from build123d import *

# Parameters (mm, degrees)
SKETCH003_R             = 23.15
PAD002_DEPTH            = 5
SKETCH004_R             = 25
PAD003_DEPTH            = 3
CHAMFER002_SIZE         = 2
SKETCH005_R             = 22
POCKET001_DEPTH         = 6
CHAMFER003_SIZE         = 2
SKETCH006_R             = 2.775
SKETCH006_R_2           = 3.5
POCKET002_DEPTH         = 5
BODY001_PLACEMENT_ANGLE = 180


with BuildPart() as part:
    # Sketch003 → Pad002 (new body)
    with BuildSketch(Plane.XY):
        Circle(SKETCH003_R)
    extrude(amount=PAD002_DEPTH)

    # Sketch004 (on Face3 of Pad002) → Pad003 (join)
    with BuildSketch(Plane.XY.offset(5)):
        Circle(SKETCH004_R)
    extrude(amount=PAD003_DEPTH)

    # Chamfer002
    chamfer002_edges = [part.edges().sort_by_distance(p)[0] for p in [
        (-25, 0, 8),
    ]]
    chamfer(chamfer002_edges, length=CHAMFER002_SIZE)

    # Sketch005 (on Face6 of Chamfer002) → Pocket001 (cut)
    with BuildSketch(Plane(origin=(0, 0, 0), x_dir=(1, 0, 0), z_dir=(0, 0, -1))):
        Circle(SKETCH005_R)
    extrude(amount=-POCKET001_DEPTH, mode=Mode.SUBTRACT)

    # Chamfer003
    chamfer003_edges = [part.edges().sort_by_distance(p)[0] for p in [
        (-22, 0, 6),
    ]]
    chamfer(chamfer003_edges, length=CHAMFER003_SIZE)

    # Sketch006 (on Face9 of Chamfer003) → Pocket002 (cut)
    with BuildSketch(Plane.XY.offset(8)):
        with Locations((0, 10)):
            Circle(SKETCH006_R)
        with Locations((0, -10)):
            Circle(SKETCH006_R_2)
    extrude(amount=-POCKET002_DEPTH, mode=Mode.SUBTRACT)


with BuildPart() as part_1:
    # Body001 placement: moved
    add(part.part.moved(Location((0, 0, -195))).rotate(Axis((0, 0, -195), (0, 1, 0)), BODY001_PLACEMENT_ANGLE))


solid = part_1.part
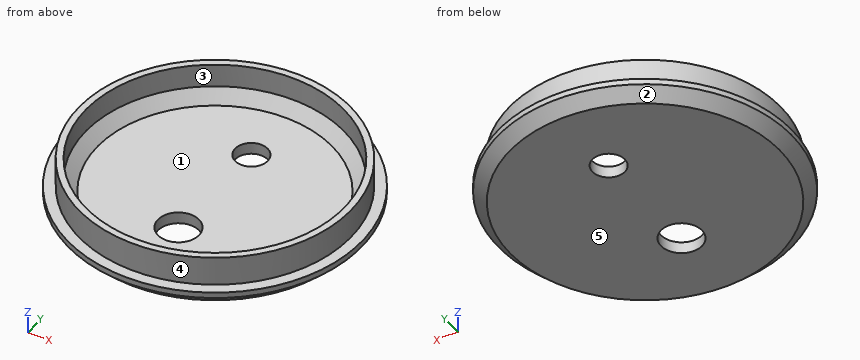
For this review, take the finished solid that the model builds, in its own axes (mm). Face numbers are marked on the shaded views. A direction names the side the tool comes from. Round coordinates to 2 decimals unless told otherwise and drop trailing zeros. Order: outer loops, then holes, each group sorted by start corner. A loop starts at its lowest first (then second) coordinate and runs counter-clockwise, first axis right, second up. Notation, with made-up numbers: (-38.5, 55.25) -> (-27.5, 55.25) arc R9 cw to (-27.5, 62.25) -> close; hole circle Ø10 at (-4.75, 88.25). An arc over 180 degrees is marked (long way). Put each result on its own line as item: value.
Q1. Add section C-C on z = -202. Write out the cut boundary in (x, y) (3 decimals).
Check result:
outline: circle Ø48 at (0, 0); hole circle Ø7 at (0, -10); hole circle Ø5.55 at (0, 10)
Q2. For probe 1 along Y at (x, z) = (0, -201.45) (3 decimals); probe 2 along Y at (x, z) = (0, -196.6); probe 3 along Y at (x, z) = (-12, -199.25), list the stretches that pass through material, from the lowest coordinate up. Write a range as [from, to].
Check result:
probe 1: [-24.55, -13.5], [-6.5, 7.225], [12.775, 24.55]
probe 2: [-23.15, -22], [22, 23.15]
probe 3: [-19.8, -18.14], [18.14, 19.8]
Q3. Insertion check: pin 1 Ø3 at (y, z) = (-1, -196.5) entering from -X; pin 2 Ø1.5 at (y, z) = (-15, -197) entering from -X; pin 3 Ø4 at (x, y) = (11, 8.5) entering from +Z. Each pin has a flat end and moves straight along its axis. Give the tip position at first contact, or say it passes through.
Check result:
pin 1: x = -23.15
pin 2: x = -18.24
pin 3: z = -201
Q4. Add section A-A on x = 0. Write out the cut boundary in (y, z) (3 decimals).
Check result:
outline: (-25, -201) -> (-23, -203) -> (-13.5, -203) -> (-13.5, -201) -> (-20, -201) -> (-22, -199) -> (-22, -195) -> (-23.15, -195) -> (-23.15, -200) -> (-25, -200) -> close; (-6.5, -203) -> (7.225, -203) -> (7.225, -201) -> (-6.5, -201) -> close; (12.775, -203) -> (23, -203) -> (25, -201) -> (25, -200) -> (23.15, -200) -> (23.15, -195) -> (22, -195) -> (22, -199) -> (20, -201) -> (12.775, -201) -> close
Q5. Add section D-D on z = -198. Write out the cut boundary in (x, y).
Check result:
outline: circle Ø46.3 at (0, 0); hole circle Ø44 at (0, 0)
Q6. Add section B-B on y = 0. Write out the cut boundary in (x, z), plus the area to 4 significant figures.
Check result:
outline: (-25, -201) -> (-23, -203) -> (23, -203) -> (25, -201) -> (25, -200) -> (23.15, -200) -> (23.15, -195) -> (22, -195) -> (22, -199) -> (20, -201) -> (-20, -201) -> (-22, -199) -> (-22, -195) -> (-23.15, -195) -> (-23.15, -200) -> (-25, -200) -> close
area: 117.5 mm2
Q7. Machinability: for the marked faces 1 and 2, which of the approach directions +Z, -Z, +X, -X, +Y, -Y give a long, thin tool a straight path to every point of the face, cutting with its end or side? Answer none if there is none.
Check result:
face 1: +Z
face 2: -Z
Q8. Mouldability with a two-part tool opening along X and no side actions: class the marked faces 3, 4 and 5 as pulls with the +X half, pulls with the -X half, needs draft (parallel to the pull), parting line crosses it, or undercut.
Check result:
face 3: undercut
face 4: parting line crosses it
face 5: needs draft
